Work out the finished part from the listing and answer in its coordinate system (mm). A direction names the side the tool comes from. Coordinates: 2 decimals unless noted, no trailing zeros. Order: outer loops, then holes, each group sorted by start corner. A loop starts at its lowest first (then second) coordinate and runs counter-clockwise, first axis right, second up. Notation, with made-up numbers: (12.5, -40) - (33.5, -40) arc R12 cw to (33.5, -18) - close; hole circle Ø1 at (43, 27). An arc over 180 degrees is marked (long way). Answer as a JSON object with one key per item and string values. Group by question number.
1) Each of these flat-tipped pins is pushed along its axis until it touches: P1, Ø1.6, axis at x = 19.5, y = -4, coming from the -Z side; P2, Ø4, axis at x = 19, z = 7.5, coming from the +Y side; P3, Ø3.5, axis at x = 4.27, y = -3.81, coming from the +Z side; P4, Ø1.9, axis at x = 27.13, y = -3.81, coming from the +Z side. Where does it stop, or does it pass through?
2) Section D-D (z = 4) is taken. Give the vertices of the cut face in (x, y).
3) Find the intervals of material crossed by line 1 along X through (y, z) = (-4.75, 7.75); line 2 along Z through (x, y) = (5.5, -3.75); line 3 along Y through (x, z) = (26, -1.5), in increasing order.
4) The mould has two halves that part along Z. Classify faces 3 (the face through (7.3, -3.8, 8.2)), 4 (the face through (1.857, -3.704, -0.939)), 5 (the face through (6, -4, -1.905)): released by +Z, released by -Z, zero draft, split by the parting line, or undercut.
5) Section A-A (z = 7.75) is taken. Give the vertices of the cut face in (x, y), plus the area to 3 significant figures.
6) Section B-B (x = 7.62) is taken. Give the vertices of the cut face in (y, z).
7) A tool of negligible diameter and unlimited length cuts with its end or side. For faces 1 (the face through (19, -2, -1.905)), 2 (the face through (14.19, -3.09, -0.94)), from which of +Z, -Z, +X, -X, +Y, -Y can it reach the whole face along a straight path? Write none if from no direction.
8) Section C-C (x = 4.5) is taken. Give the vertices of the cut face in (y, z) (3 decimals), plus the area to 3 significant figures.
from build123d import *

# Parameters (mm, degrees)
F0_R     = 2.919268
F0_R_2   = 2.504925
F1_DEPTH = 7.62
F2_R     = 2.413
F2_R_2   = 1.5875
F3_DEPTH = 1.905


with BuildPart() as f1:
    # F0 (on Front) → F1 (new body)
    with BuildSketch(Plane.XZ):
        Polygon((30.479431, 8.89), (0, 9.076191), (0, 0), (30.479431, 0), align=None)
        with Locations((7.62, 5.715)):
            Circle(F0_R, mode=Mode.SUBTRACT)
        with Locations((15.24, 5.715)):
            Circle(F0_R, mode=Mode.SUBTRACT)
        with Locations((22.86, 5.715)):
            Circle(F0_R, mode=Mode.SUBTRACT)
        with Locations((15.24, 5.715)):
            Circle(F0_R)
        with Locations((15.24, 5.715)):
            Circle(F0_R_2, mode=Mode.SUBTRACT)
        with Locations((22.86, 5.715)):
            Circle(F0_R)
        with Locations((22.86, 5.715)):
            Circle(F0_R_2, mode=Mode.SUBTRACT)
        with Locations((7.62, 5.715)):
            Circle(F0_R)
        with Locations((7.62, 5.715)):
            Circle(F0_R_2, mode=Mode.SUBTRACT)
    extrude(amount=F1_DEPTH)

    # F2 (on Top) → F3 (join)
    with BuildSketch(Plane.XY):
        with Locations((4.267945, -3.81)):
            Circle(F2_R)
        with Locations((4.267945, -3.81)):
            Circle(F2_R_2, mode=Mode.SUBTRACT)
        with Locations((11.887945, -3.81)):
            Circle(F2_R)
        with Locations((11.887945, -3.81)):
            Circle(F2_R_2, mode=Mode.SUBTRACT)
        with Locations((19.507945, -3.81)):
            Circle(F2_R)
        with Locations((19.507945, -3.81)):
            Circle(F2_R_2, mode=Mode.SUBTRACT)
        with Locations((27.127945, -3.81)):
            Circle(F2_R)
        with Locations((27.127945, -3.81)):
            Circle(F2_R_2, mode=Mode.SUBTRACT)
    extrude(amount=-F3_DEPTH)


solid = f1.part
Report:
{
 "1": {"P1": "stops at z = 0", "P2": "stops at y = 0", "P3": "stops at z = 9.06", "P4": "stops at z = 8.92"},
 "2": {"outline": "(0, -7.62) - (5.79, -7.62) - (5.79, 0) - (0, 0) - close; (9.45, -7.62) - (13.41, -7.62) - (13.41, 0) - (9.45, 0) - close; (17.07, -7.62) - (21.03, -7.62) - (21.03, 0) - (17.07, 0) - close; (24.69, -7.62) - (30.48, -7.62) - (30.48, 0) - (24.69, 0) - close"},
 "3": {"line 1": "x = 0 to 6.16, 9.08 to 13.78, 16.7 to 21.4, 24.32 to 30.48", "line 2": "z = 0 to 4.38, 7.05 to 9.04", "line 3": "y = -5.94 to -4.93, -2.69 to -1.68"},
 "4": {"face 3": "undercut", "face 4": "zero draft", "face 5": "released by -Z"},
 "5": {"outline": "(0, -7.62) - (6.16, -7.62) - (6.16, 0) - (0, 0) - close; (9.08, -7.62) - (13.78, -7.62) - (13.78, 0) - (9.08, 0) - close; (16.7, -7.62) - (21.4, -7.62) - (21.4, 0) - (16.7, 0) - close; (24.32, -7.62) - (30.48, -7.62) - (30.48, 0) - (24.32, 0) - close", "area": "165 mm²"},
 "6": {"outline": "(-7.62, 0) - (0, 0) - (0, 3.21) - (-7.62, 3.21) - close; (-7.62, 8.22) - (0, 8.22) - (0, 9.03) - (-7.62, 9.03) - close"},
 "7": {"face 1": "-Z, +X, -X, +Y, -Y", "face 2": "-Z"},
 "8": {"outline": "(-7.62, 0) - (-6.212, 0) - (-6.212, -1.905) - (-5.38, -1.905) - (-5.38, 0) - (-2.24, 0) - (-2.24, -1.905) - (-1.408, -1.905) - (-1.408, 0) - (0, 0) - (0, 9.049) - (-7.62, 9.049) - close", "area": "72.1 mm²"}
}
